```python
from build123d import *

# Parameters (mm, degrees)
SKETCH_1_R              = 1.75
EXTRUDE_1_DEPTH         = 3
EXTRUDE_2586_DEPTH      = 11
EXTRUDE_2586_DEPTH_BACK = 3
FILLET1_R               = 10


with BuildPart() as part:
    # Эскиз1 → Бобышка-Вытянуть1 (new body)
    with BuildSketch(Plane(origin=(0, 0, 0), x_dir=(1, 0, 0), z_dir=(0, 1, 0))):
        with BuildLine():
            Line((0, 48), (0, 52))
            ThreePointArc((0, 52), (6.283445482, 51.618972412), (12.474807654, 50.481473572))
            ThreePointArc((12.474807654, 50.481473572), (14.921144436, 55.582006519), (20.5212086, 56.381557247))
            ThreePointArc((20.5212086, 56.381557247), (38.567256581, 45.962666587), (51.961524227, 30))
            ThreePointArc((51.961524227, 30), (49.765371804, 21.803847577), (41.569219382, 24))
            ThreePointArc((41.569219382, 24), (24, 41.569219382), (0, 48))
        make_face()
        with Locations(Location((34.710530923, 41.366399928, 0), (0, 0, 270))):
            Circle(SKETCH_1_R, mode=Mode.SUBTRACT)
        with Locations(Location((18.46908774, 50.743401522, 0), (0, 0, 270))):
            Circle(SKETCH_1_R, mode=Mode.SUBTRACT)
        with Locations(Location((46.765371804, 27, 0), (0, 0, 270))):
            Circle(SKETCH_1_R, mode=Mode.SUBTRACT)
    extrude(amount=EXTRUDE_1_DEPTH)

    # Эскиз2 → Extrude 2586 (add, two sides: drawn at the far end of the back side and taken through both)
    with BuildSketch(Plane(origin=(0, 3, 0), x_dir=(1, 0, 0), z_dir=(0, 1, 0)).offset(-EXTRUDE_2586_DEPTH_BACK)):
        with BuildLine():
            Line((49.302845964, -19.419222091), (49.302845964, -18.005008529))
            Line((49.302845964, -18.005008529), (47.888632402, -18.005008529))
            Line((47.888632402, -18.005008529), (47.888632402, -16.590794966))
            Line((47.888632402, -16.590794966), (46.474418839, -16.590794966))
            Line((46.474418839, -16.590794966), (46.474418839, -15.176581404))
            Line((46.474418839, -15.176581404), (45.060205277, -15.176581404))
            Line((45.060205277, -15.176581404), (45.060205277, -13.762367842))
            Line((45.060205277, -13.762367842), (43.645991715, -13.762367842))
            Line((43.645991715, -13.762367842), (43.645991715, -12.348154279))
            Line((43.645991715, -12.348154279), (42.231778152, -12.348154279))
            ThreePointArc((42.231778152, -12.348154279), (35.208797113, 26.388266443), (0, 44))
            Line((0, 44), (0, 48))
            ThreePointArc((0, 48), (37.676689525, 29.73999103), (46.687683687, -11.147205565))
            Line((46.687683687, -11.147205565), (52.131273089, -16.590794966))
            Line((52.131273089, -16.590794966), (49.302845964, -19.419222091))
        make_face()
    extrude(amount=EXTRUDE_2586_DEPTH + EXTRUDE_2586_DEPTH_BACK)

    # Fillet1
    fillet1_edges = [part.edges().sort_by_distance(p)[0] for p in [
        (41.569219382, 1.5, -24),
    ]]
    fillet(fillet1_edges, radius=FILLET1_R)


solid = part.part
```
Design review of the part built by this model. Coordinates are the model's own, in mm. A direction names the side the tool comes from. Round coordinates to 2 decimals unless told otherwise and drop trailing zeros. Write each loop counter-clockwise with the first axis right and the second up, starting at its lowest first coordinate (ties: lowest second). Pieces come first, ordered by that corner, then holes. Notation, with made-up numbers: (74.5, -9) -> (128.5, -9) arc R4 cw to (128.5, -4) -> close; hole circle Ø6 at (-17.5, 83.5). An arc over 180 degrees is marked (long way). Write item = value, one per line. Start each with the question number.
1) Wall thickness on probe 1 along X at (y, z) = (0.85, -27); probe 2 along Z at (x, y) = (16.5, 7); probe 3 along Y at (x, z) = (44, -35): over which ranges is each line inside the solid? List them lowest first. Write a range as from..to.
2) Take a section at C-C, the plane y = 2.25. Count the separate pieces of the cut face and the enclosed holes in it, plus the area to 3 significant figures.
3) Take a section at B-B, the plane x = 10. State the section outline as (y, z) points.
4) Clearance check with flat-ended pins moving along their axes: pin 1 (2 mm diameter, centred on y = 3, z = -47, fed in from +X); pin 2 (3 mm diameter, centred on x = 34.71, z = -41.37, fed in from -Y); pin 3 (1 mm diameter, centred on x = 26, y = 11, fed in from +Z); pin 4 (4.5 mm diameter, centred on x = 46.77, z = -27, fed in from +Y). State where each tip first meets the part, or that it passes through.
5) Take a section at D-D, the plane z = -46. State the section outline as (x, y) points.
6) Mouldability with a two-part tool opening along X and no side actions: class faces 4 (the face through (50.737, 6.902, 17.985)), 5 (the face through (32, 3, -41)), 6 (the face through (6.2, 1.48, -51.63)) as +X half, -X half, draft (parallel to the pull), parting line (faces both ways), or undercut.
7) Tool access review of faces 1 (the face through (49.37, 6.9, 13.83)), 2 (the face through (47.889, 7, 17)), 3 (the face through (37.3, 8.46, -30.21)): name each direction out of +Z, -Z, +X, -X, +Y, -Y from which nothing blocks a thin tool from reaching the whole face with its end or side.
8) Take a section at A-A, the plane z = -27. State the section outline as (x, y) points, plus the area to 3 significant figures.
Results list:
q1.probe_1 = 34.74..45.02, 48.52..52.77
q1.probe_2 = -45.07..-40.79
q1.probe_3 = 0..3
q2.separate_pieces = 1
q2.enclosed_holes = 3
q2.area = 977 mm²
q3.outline = (0, -51.03) -> (3, -51.03) -> (3, -46.95) -> (14, -46.95) -> (14, -42.85) -> (0, -42.85) -> close
q4.pin_1 = 38.52
q4.pin_2 = through
q4.pin_3 = -35.12
q4.pin_4 = 3
q5.outline = (0, 0) -> (38.52, 0) -> (38.52, 3) -> (13.71, 3) -> (13.71, 14) -> (0, 14) -> close
q6.face_4 = +X half
q6.face_5 = draft
q6.face_6 = undercut
q7.face_1 = +X, +Y, -Y
q7.face_2 = +Z, -X, +Y, -Y
q7.face_3 = +X, +Y
q8.outline = (34.74, 0) -> (45.02, 0) -> (45.02, 3) -> (39.69, 3) -> (39.69, 14) -> (34.74, 14) -> close; (48.52, 0) -> (52.77, 0) -> (52.77, 3) -> (48.52, 3) -> close
q8.area = 98.0 mm²
